For this review, use the dimensioned drawing (mm, ordinates from the lowest corner) and the shaded views. A direction names the side the tool comes from. Give positions to 0.01 mm unless a question says otherwise; leave off trailing zeros. Loops run counter-clockwise (first coordinate to the right, second up) from the corner with the lowest first, then second, coordinate; pieces in that order, holes last. Notation, with made-up numbers: M 1,71.25 L 51,71.25 A11 cw 51,80.25 Z; hole C -26,65.25 d7. An arc over 180 degrees is marked long. Use a Markdown table: item, result. Add a question column.
(1) Insertion check: pin 1 Ø10 at (x, z) = (48, 31.5) entering from -Y; pin 2 Ø5 at (x, z) = (97.5, 37.5) entering from -Y (1 decimal); pin 3 Ø6 at (y, z) = (126.5, 22) entering from -X; pin 4 Ø10 at (x, y) = (79.5, 65.5) entering from +Z. Each pin has a flat end and moves straight along its axis. Give the tip position at first contact, or say it passes through.
(2) Add section C-C, the plane z = 29.5. Give the boundary of the cut face in (x, y).
(3) Add section A-A, the plane y = 70.5. Give the boundary of the cut face in (x, z), then the cut area to 3 significant figures.
(4) Add section B-B, the plane x = 70.5. State how many separate pieces and enclosed holes the cut face has, then the cut area to 3 significant figures.
(5) For probe 1 along Y at (x, z) = (70, 28); probe 2 along X at (y, z) = (70.5, 17.5); probe 3 along Y at (x, z) = (74, 32.5) (1 decimal), list the stretches that pass through material, from the lowest coordinate up.
(6) For the marked faces 4 and 5, list the 3-axis set-ups (+Z, -Z, +X, -X, +Y, -Y) from which the entire face can be reached by the end or side of a thin tool; tool diameter is ignored.
(7) Draft analysis for pull direction Y (two halves, no side actions). For the marked faces 1, 2 and 3, state which applies: pulls with the +Y half, pulls with the -Y half, needs draft (parallel to the pull), parting line crosses it, or undercut.
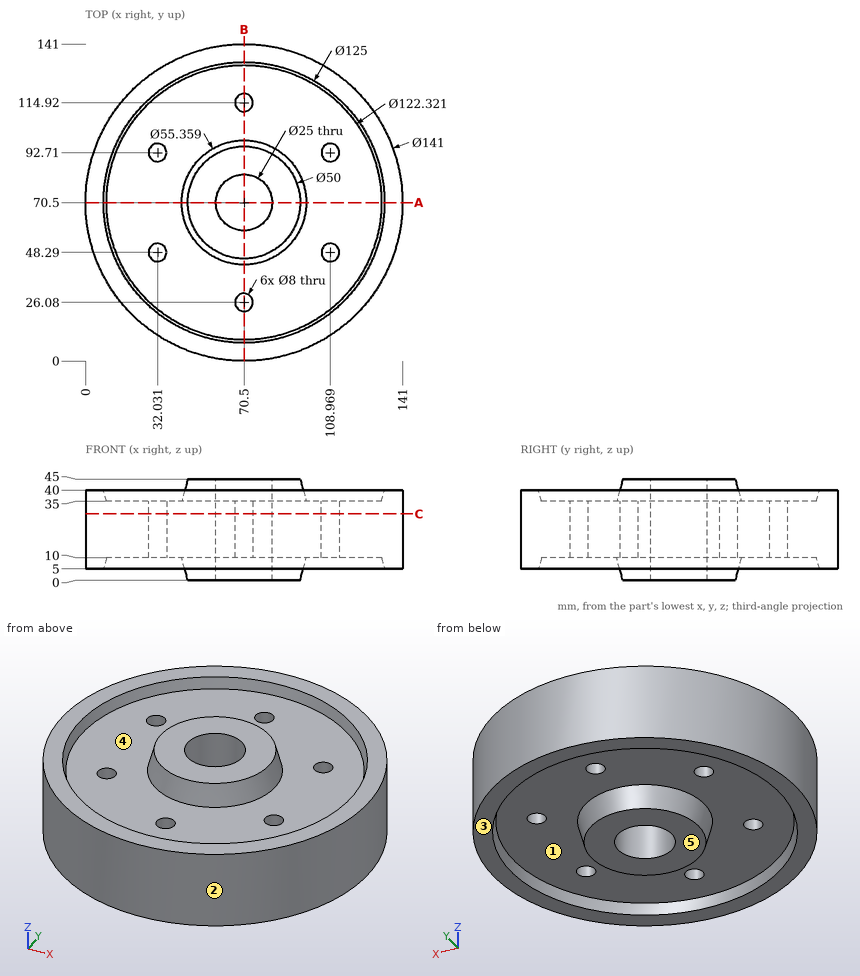
Established:
| question | item | result |
|---|---|---|
| 1 | pin 1 | y = 2.21 |
| 1 | pin 2 | y = 4.4 |
| 1 | pin 3 | x = 24.01 |
| 1 | pin 4 | z = 45 |
| 2 | outline | C 70.5,70.5 d141; hole C 32.03,48.29 d8; hole C 32.03,92.71 d8; hole C 70.5,70.5 d25; hole C 70.5,26.08 d8; hole C 70.5,114.92 d8; hole C 108.97,48.29 d8; hole C 108.97,92.71 d8 |
| 3 | outline | M 0,5 L 8,5 L 9.34,10 L 42.82,10 L 45.5,0 L 58,0 L 58,45 L 45.5,45 L 42.82,35 L 9.34,35 L 8,40 L 0,40 Z; M 83,0 L 95.5,0 L 98.18,10 L 131.66,10 L 133,5 L 141,5 L 141,40 L 133,40 L 131.66,35 L 98.18,35 L 95.5,45 L 83,45 Z |
| 3 | area | 3,630 mm^2 |
| 4 | separate pieces | 4 |
| 4 | enclosed holes | 0 |
| 4 | area | 3,230 mm^2 |
| 5 | probe 1 | 0 to 22.11, 30.05 to 58.01, 82.99 to 110.95, 118.89 to 141 |
| 5 | probe 2 | 0 to 58, 83 to 141 |
| 5 | probe 3 | 0.1 to 24.1, 28 to 58.5, 82.5 to 113, 116.9 to 140.9 |
| 6 | face 4 | +Z |
| 6 | face 5 | -Z, +X, -X, +Y, -Y |
| 7 | face 1 | undercut |
| 7 | face 2 | parting line crosses it |
| 7 | face 3 | needs draft |
